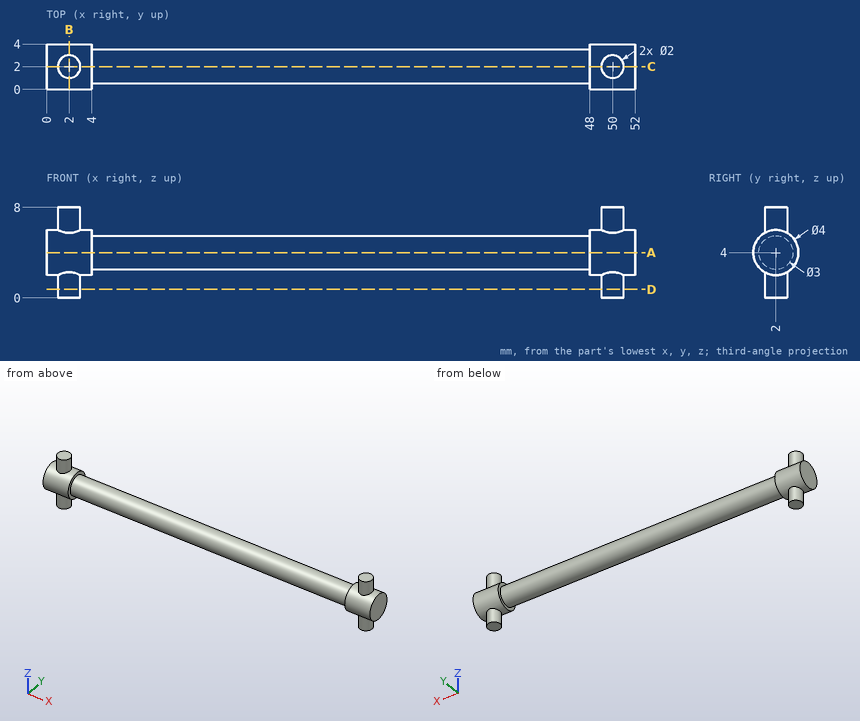
Geometry: see drawing. Coordinates: mm, zero at the bounding-box minimum. Round coordinates to 2 decimals unless told otherwise and drop trailing zeros. Write each loop counter-clockwise with the first axis right and the second up, starting at its lowest first coordinate (ties: lowest second). Pieces come first, ordered by that corner, then holes.
1) Cut plane C-C (y = 2). Return the cut outline in (x, z).
2) Cut plane D-D (z = 0.75). Return the cut outline in (x, y), then the cut area to 3 significant figures.
3) Contact query for a flat-ended pin moving along its axis: P1, Ø2, axis at x = 27.5, z = 6, coming from the +Y side. Output: stop coordinate, or through.
4) Cut plane B-B (x = 2). Return the cut outline in (y, z), then the cut area to 3 significant figures.
5) Cut plane A-A (z = 4). Return the cut outline in (x, y).
6) Ray query, L1, parallel to X at y = 3, z = 5.5; L2, parallel to Z at x = 17.5, y = 1.95; L3, parallel to X at y = 2.9, z = 7.5. Return the intervals inside material, ascending.
Geometry says:
1. outline: (0, 2) - (1, 2) - (1, 0) - (3, 0) - (3, 2) - (4, 2) - (4, 2.5) - (48, 2.5) - (48, 2) - (49, 2) - (49, 0) - (51, 0) - (51, 2) - (52, 2) - (52, 6) - (51, 6) - (51, 8) - (49, 8) - (49, 6) - (48, 6) - (48, 5.5) - (4, 5.5) - (4, 6) - (3, 6) - (3, 8) - (1, 8) - (1, 6) - (0, 6) - close
2. outline: circle Ø2 at (2, 2); circle Ø2 at (50, 2)
2. area: 6.28 mm2
3. P1: stops at y = 3.12
4. outline: (1, 0) - (3, 0) - (3, 2.27) arc R2 ccw to (3, 5.73) - (3, 8) - (1, 8) - (1, 5.73) arc R2 ccw to (1, 2.27) - close
4. area: 20.9 mm2
5. outline: (0, 0) - (4, 0) - (4, 0.5) - (48, 0.5) - (48, 0) - (52, 0) - (52, 4) - (48, 4) - (48, 3.5) - (4, 3.5) - (4, 4) - (0, 4) - close
6. L1: x = 0 to 4, 48 to 52
6. L2: z = 2.5 to 5.5
6. L3: x = 1.56 to 2.44, 49.56 to 50.44
